Could you check a few things on this model? Use its own coordinates, in mm. A direction names the side the tool comes from. Round coordinates to 2 decimals unless told otherwise and drop trailing zeros. Loops run counter-clockwise (first coordinate to the right, second up) from the corner with the lowest first, then second, coordinate; pieces in that order, holes last. Notation, with made-up numbers: (10.25, -15) -> (29.25, -15) arc R8 cw to (29.25, -5) -> close; hole circle Ø10 at (59, 9.25). An arc over 180 degrees is marked (long way). Put each result on its own line as item: value. Start each with the question number.
1. Imagine slicing it at B-B, the plane y = -5.5. Please give me the cut outline in (x, z) (3 decimals).
2. Imagine slicing it at C-C, the plane z = 1.5. Count the separate pieces of the cut face and the enclosed holes in it, and give its area (3 significant figures).
3. Which directions (+Z, -Z, +X, -X, +Y, -Y) give clear straight access to the entire face, cutting with the end or side of a thin tool? Please do faces 4 (the cylindrical face through (-2.848, 5.374, 10.771)), 5 (the cylindrical face through (0, 5, -7)), 6 (the flat face through (9, -7, 4.7)), 7 (the flat face through (9, -5, -0.5)).
4. I need wall thicknesses on line 1 (Y direction, x = 11, z = 9.5); line 2 (Z direction, x = 0, y = -5.25) (3 decimals); line 3 (Y direction, x = 11, z = 2.7). Which ranges of each line are inside material? Lowest first, please. Write a range as [from, to].
5. I'm going to push flat-ended pins straight in: P1, Ø8.5, axis at x = 11, y = -5.5, coming from the -Z side; P2, Ø10, axis at x = 7.5, y = 0, coming from the +Z side; P3, Ø13.5, axis at x = 1, z = 2.5, coming from the +Y side; P4, Ø12, axis at y = 8, z = 8, coming from the -X side. Where does each tip first touch, or does it pass through?
6. If we mould it in two halves opening along Y, with no side actions, what happens to faces 1 (the flat face through (0, 11, -12)), 2 (the flat face through (8, -5, 0.5)), 3 (the cylindrical face through (7.253, -5.637, 7.92))? For each: pulls with the +Y half, pulls with the -Y half, needs draft (parallel to the pull), parting line crosses it, or undercut.
7. Imagine slicing it at A-A, the plane y = 3.5. Please give me the cut outline in (x, z), and give its area (3 significant figures).
```python
from build123d import *

# Parameters (mm, degrees)
SKETCH1_R                   = 15
BOSS_EXTRUDE1_DEPTH         = 11
SKETCH2_R                   = 7
CUT_EXTRUDE1_DEPTH          = 23
SKETCH3_R                   = 17
CUT_EXTRUDE2_DEPTH          = 11
CUT_EXTRUDE3_DEPTH          = 11
SKETCH5_W                   = 16.165630516
SKETCH5_H                   = 1
CUT_EXTRUDE4_DEPTH          = 21
SKETCH6_R                   = 2
CUT_EXTRUDE5_DEPTH          = 21
CUT_EXTRUDE6_START          = -4.2
SKETCH7_R                   = 3.75
CUT_EXTRUDE6_DEPTH          = 21
M4_TAPPED_HOLE1_D           = 3.3
M4_TAPPED_HOLE1_DEPTH       = 20.1
M4_TAPPED_HOLE1_TIP         = 0.991420021
CHAMFER1_SIZE               = 0.4
SKETCH10_R                  = 0.3
CHAMFER2_SIZE               = 0.1
Y_KSEKLIK_EKSTR_ZYON1_DEPTH = 11


with BuildPart() as part:
    # Sketch1 → Boss-Extrude1 (new, symmetric)
    with BuildSketch(Plane(origin=(0, 0, 0), x_dir=(1, 0, 0), z_dir=(0, 1, 0))):
        with Locations(Location((0, 0, 0), (0, 0, 270))):
            Circle(SKETCH1_R)
    extrude(amount=BOSS_EXTRUDE1_DEPTH, both=True)

    # Sketch2 → Cut-Extrude1 (cut)
    with BuildSketch(Plane(origin=(0, 11, 0), x_dir=(1, 0, 0), z_dir=(0, 1, 0))):
        with Locations(Location((0, 0, 0), (0, 0, 270))):
            Circle(SKETCH2_R)
    extrude(amount=-CUT_EXTRUDE1_DEPTH, mode=Mode.SUBTRACT)

    # Sketch3 → Cut-Extrude2 (cut)
    with BuildSketch(Plane(origin=(0, 11, 0), x_dir=(1, 0, 0), z_dir=(0, 1, 0))):
        with Locations((16, 0)):
            Circle(SKETCH3_R)
    extrude(amount=-CUT_EXTRUDE2_DEPTH, mode=Mode.SUBTRACT)

    # Sketch4 → Cut-Extrude3 (cut)
    with BuildSketch(Plane(origin=(0, 11, 0), x_dir=(1, 0, 0), z_dir=(0, 1, 0))):
        with BuildLine():
            ThreePointArc((-6, 13.747727085), (-15, 0), (-6, -13.747727085))
            ThreePointArc((-6, -13.747727085), (-2.808871931, -10.72353208), (-0.5, -6.982120022))
            ThreePointArc((-0.5, -6.982120022), (-7, 0), (-0.5, 6.982120022))
            ThreePointArc((-0.5, 6.982120022), (-2.808871931, 10.72353208), (-6, 13.747727085))
        make_face()
    extrude(amount=-CUT_EXTRUDE3_DEPTH, mode=Mode.SUBTRACT)

    # Sketch5 → Cut-Extrude4 (cut)
    with BuildSketch(Plane(origin=(0, 0, 0), x_dir=(1, 0, 0), z_dir=(0, 1, 0))):
        with Locations((11.807437966, 0)):
            Rectangle(SKETCH5_W, SKETCH5_H)
    extrude(amount=-CUT_EXTRUDE4_DEPTH, mode=Mode.SUBTRACT)

    # Sketch6 → Cut-Extrude5 (cut)
    with BuildSketch(Plane.XY):
        with Locations(Location((11, -5.5, 0), (0, 0, 180))):
            Circle(SKETCH6_R)
    extrude(amount=CUT_EXTRUDE5_DEPTH, mode=Mode.SUBTRACT)

    # Sketch7 → Cut-Extrude6 (cut)
    with BuildSketch(Plane(origin=(0, 0, 0.5), x_dir=(-1, 0, 0), z_dir=(0, 0, -1)).offset(CUT_EXTRUDE6_START)):
        with Locations((-11, -5.5)):
            Circle(SKETCH7_R)
    extrude(amount=-CUT_EXTRUDE6_DEPTH, mode=Mode.SUBTRACT)

    # M4 Tapped Hole1
    with Locations(Plane.XY.offset(-0.5)):
        with Locations((11, -5.5)):
            Hole(M4_TAPPED_HOLE1_D / 2, depth=M4_TAPPED_HOLE1_DEPTH)
            with Locations((0, 0, -(M4_TAPPED_HOLE1_DEPTH + M4_TAPPED_HOLE1_TIP / 2))):  # 118° drill point
                Cone(0, M4_TAPPED_HOLE1_D / 2, M4_TAPPED_HOLE1_TIP, mode=Mode.SUBTRACT)

    # Chamfer1
    chamfer1_edges = [part.edges().sort_by_distance(p)[0] for p in [
        (0, 11, -7),
        (2.808871931, 11, 10.72353208),
        (2.808871931, 11, -10.72353208),
        (0, 11, 7),
        (-2.808871931, 11, -10.72353208),
        (-2.808871931, 11, 10.72353208),
    ]]
    chamfer(chamfer1_edges, length=CHAMFER1_SIZE)

    # Sketch10 → Cut-Revolve1 (revolve, cut)
    with BuildSketch(Plane(origin=(0, 0, 0), x_dir=(0, 0, -1), z_dir=(1, 0, 0))):
        with Locations((15, 0.3)):
            Circle(SKETCH10_R)
    revolve(axis=Axis((0, 3.360414074, 0), (0, -1, 0)), mode=Mode.SUBTRACT)

    # Chamfer2
    chamfer2_edges = [part.edges().sort_by_distance(p)[0] for p in [
        (-15, -11, 0),
    ]]
    chamfer(chamfer2_edges, length=CHAMFER2_SIZE)

    # Çizim1 → Yükseklik-Ekstrüzyon1 (add)
    with BuildSketch(Plane(origin=(0, 0, 0), x_dir=(1, 0, 0), z_dir=(0, 1, 0))):
        with BuildLine():
            Line((6.982120022, 0.5), (3.135382752, 0.5))
            ThreePointArc((3.135382752, 0.5), (-3.175, 0), (3.135382752, -0.5))
            Line((3.135382752, -0.5), (6.982120022, -0.5))
            ThreePointArc((6.982120022, -0.5), (-7, 0), (6.982120022, 0.5))
        make_face()
    extrude(amount=-Y_KSEKLIK_EKSTR_ZYON1_DEPTH)


solid = part.part
```
Entries:
1. outline: (3.135, -0.5) arc R3.175 cw (long way) to (3.135, 0.5) -> (9, 0.5) -> (9, 4.7) -> (7.25, 4.7) -> (7.25, 13.132) arc R15 ccw (long way) to (9.35, -11.729) -> (9.35, -0.5) -> close; (12.65, -8.061) arc R15 ccw to (14.992, -0.5) -> (12.65, -0.5) -> close; (13, 0.5) -> (14.992, 0.5) arc R15 ccw to (14.245, 4.7) -> (13, 4.7) -> close
2. separate pieces: 2
2. enclosed holes: 1
2. area: 254 mm^2
3. face 4: -X, +Y
3. face 5: +Y
3. face 6: +Z
3. face 7: +X, +Y, -Y
4. line 1: [-11, -9.25], [-1.75, 0]
4. line 2: [-15, -3.175], [3.175, 15]
4. line 3: [-11, -7.5], [-3.5, 0]
5. P1: z = -13.4
5. P2: z = 14.79
5. P3: y = 11
5. P4: x = -6
6. face 1: pulls with the +Y half
6. face 2: needs draft
6. face 3: undercut
7. outline: (-6, -13.75) arc R15 ccw to (6, -13.75) arc R17 cw to (0.5, -6.98) arc R7 cw to (-0.5, -6.98) arc R17 cw to start; (-6, 13.75) arc R17 cw to (-0.5, 6.98) arc R7 cw to (0.5, 6.98) arc R17 cw to (6, 13.75) arc R15 ccw to start
7. area: 94.9 mm^2
